```python
from build123d import *

# Parameters (mm, degrees)
CUT_EXTRUDE1_DEPTH = 6


with BuildPart() as part:
    # Sketch1 → Revolve1 (revolve)
    with BuildSketch(Plane(origin=(0, 0, 0), x_dir=(0, 0, -1), z_dir=(1, 0, 0))):
        Polygon((0, 0), (0, 11.55405041), (-1.5, 13.05405041), (-10.5, 13.335), (-12, 11.835), (-12, 0), align=None)
    revolve(axis=Axis((0, 0, 0), (0, 0, 1)))

    # Sketch2 → Cut-Extrude1 (cut)
    with BuildSketch(Plane.XY.offset(12)):
        Polygon((0, -8.313843876), (7.2, -4.156921938), (7.2, 4.156921938), (0, 8.313843876), (-7.2, 4.156921938), (-7.2, -4.156921938), align=None)
    extrude(amount=-CUT_EXTRUDE1_DEPTH, mode=Mode.SUBTRACT)


solid = part.part
```
Read the model definition and answer for the solid it produces. Units are mm, in the model's axes. A direction names the side the tool comes from. Give positions to 0.01 mm unless a question says otherwise; leave off trailing zeros. Write each loop counter-clockwise with the first axis right and the second up, starting at its lowest first coordinate (ties: lowest second). Pieces come first, ordered by that corner, then holes. Notation, with made-up numbers: M 89,64.5 L 97,64.5 A25 ccw 97,79.5 Z; hole C 19.25,-36 d2. An arc over 180 degrees is marked long. Put each result on its own line as item: value. Start each with the question number.
1. The part is cut by section C-C, the plane z = 3.5. Give the vertices of the cut face in (x, y).
2. Consider line 1 along Z through (x, y) = (5.75, -2); line 2 along Y through (x, z) = (3.5, 10); line 3 along X through (y, z) = (-4, 11). Determine where each line is inside the solid, lowest interval first.
3. The part is cut by section A-A, the plane z = 7.5. Give the vertices of the cut face in (x, y), and give its area (3 significant figures).
4. The part is cut by section B-B, the plane y = 0. Give the vertices of the cut face in (x, z) (3 decimals), and give its area (3 significant figures).
5. Which of the six approach directions +Z, -Z, +X, -X, +Y, -Y give full straight-line access (tool end or side, diameter ignored) to faces 1 (the flat face through (8, 0, 12)), 2 (the flat face through (0, 0, 6))?
6. Each of these flat-tipped pins is pushed along its axis until it touches: pin 1 Ø5 at (y, z) = (-7.5, 5.5) entering from -X; pin 2 Ø5 at (y, z) = (1.5, 8) entering from -X; pin 3 Ø2 at (x, y) = (3, 0) entering from +Z. Where does it stop, or does it pass through?
7. For a pull along X with two mould halves and no side action, classify faces 3 (the flat face through (-3.55, 6.264, 9.042)), 4 (the flat face through (3.65, 6.206, 9.042)), 5 (the flat face through (0, 0, 0)), 6 (the conical face through (11.708, 6.089, 6.063)) as released by +X, released by -X, zero draft, split by the parting line, or undercut.
Final values:
1. outline: C 0,0 d26.23
2. line 1: z = 0 to 6
2. line 2: y = -12.85 to -6.29, 6.29 to 12.85
2. line 3: x = -12.2 to -7.2, 7.2 to 12.2
3. outline: C 0,0 d26.48; hole M -7.2,-4.16 L 0,-8.31 L 7.2,-4.16 L 7.2,4.16 L 0,8.31 L -7.2,4.16 Z
3. area: 371 mm²
4. outline: M -13.335,10.5 L -13.054,1.5 L -11.554,0 L 11.554,0 L 13.054,1.5 L 13.335,10.5 L 11.835,12 L 7.2,12 L 7.2,6 L -7.2,6 L -7.2,12 L -11.835,12 Z
4. area: 226 mm²
5. face 1: +Z, +X, -X, +Y, -Y
5. face 2: +Z
6. pin 1: stops at x = -12.2
6. pin 2: stops at x = -13.32
6. pin 3: stops at z = 6
7. face 3: undercut
7. face 4: undercut
7. face 5: zero draft
7. face 6: split by the parting line
